Check sheet for the modelled part. Datum: model origin and axes. Units: mm. A direction names the side the tool comes from. Round coordinates to 2 decimals unless told otherwise and drop trailing zeros. Loops run counter-clockwise (first coordinate to the right, second up) from the corner with the lowest first, then second, coordinate; pieces in that order, holes last. Notation, with made-up numbers: (0.25, -32) -> (30.25, -32) arc R35 ccw to (30.25, 7) -> close; hole circle Ø2 at (42, 39). An arc over 180 degrees is marked (long way). One line per item, written item: value. Start each with the question number.
1. Go/stop test with flat-tipped pins: pin 1 (1.8 mm diameter, centred on x = 18, y = -3.5, fed in from +Z); pin 2 (10 mm diameter, centred on x = -5.5, y = 3.5, fed in from +Z); pin 3 (8 mm diameter, centred on x = 10.65, y = 0, fed in from +Z). Record where each tip stops, or that it passes through.
2. Cross-section at D-D on x = -10.65. Record the cut outline in (y, z), then the cut area to 3 significant figures.
3. Cross-section at C-C on z = 14. Record the cut outline in (x, y).
4. Material ranges on L1, parallel to Y at x = -10.65, z = -2.75; L2, parallel to Z at x = -4, y = 6.5; L3, parallel to Z at x = 13, y = 5.75, recorded low to high.
5. Set-up check for faces 4 (the face through (17, 0, 0)), 5 (the face through (-9.35, 0, 12)), 6 (the face through (-8.78, 0.14, 7.6)), 7 (the face through (-11.517, 3.905, -1.549)): record each of +Z, -Z, +X, -X, +Y, -Y from which the full face is reachable in a straight line by a thin tool's end or side.
6. Release check for a two-part mould opening along X. For faces 1 (the face through (-0.6, -0.14, -4.43)), 2 (the face through (-22, 0, 6)), 3 (the face through (4.85, 0, 8)) record: +X half, -X half, draft (parallel to the pull), parting line (faces both ways), or undercut.
from build123d import *

# Parameters (mm, degrees)
SKETCH_W        = 50
SKETCH_H        = 20
PAD_DEPTH       = 7
SKETCH001_W     = 11.6
SKETCH001_H     = 20
PAD001_DEPTH    = 1.2
SKETCH002_R     = 3.5
POCKET_DEPTH    = 8.201
SKETCH003_R     = 6
POCKET001_DEPTH = 1
CHAMFER_SIZE    = 2.49
SKETCH004_W     = 25
SKETCH004_H     = 20
PAD002_DEPTH    = 5
SKETCH005_R     = 4
POCKET002_DEPTH = 7
SKETCH006_W     = 15.65
SKETCH006_H     = 20
PAD003_DEPTH    = 10
POCKET003_DEPTH = 22.001
FILLET_R        = 2


with BuildPart() as part:
    # Sketch → Pad (new body)
    with BuildSketch(Plane.XY):
        Rectangle(SKETCH_W, SKETCH_H)
    extrude(amount=PAD_DEPTH)

    # Sketch001 (on Face6 of Pad) → Pad001 (join)
    with BuildSketch(Plane.XY.offset(7)):
        with Locations((10.65, 0)):
            Rectangle(SKETCH001_W, SKETCH001_H)
    extrude(amount=PAD001_DEPTH)

    # Sketch002 (on Face4 of Pad001) → Pocket (cut, through all)
    with BuildSketch(Plane(origin=(0, 0, 0), x_dir=(1, 0, 0), z_dir=(0, 0, -1))):
        with Locations((10.65, 0)):
            Circle(SKETCH002_R)
    extrude(amount=-POCKET_DEPTH, mode=Mode.SUBTRACT)

    # Sketch003 (on Face4 of Pocket) → Pocket001 (cut)
    with BuildSketch(Plane(origin=(0, 0, 0), x_dir=(1, 0, 0), z_dir=(0, 0, -1))):
        with Locations((10.65, 0)):
            Circle(SKETCH003_R)
    extrude(amount=-POCKET001_DEPTH, mode=Mode.SUBTRACT)

    # Chamfer
    chamfer_edges = [part.edges().sort_by_distance(p)[0] for p in [
        (7.15, 0, 1),
    ]]
    chamfer(chamfer_edges, length=CHAMFER_SIZE)

    # Sketch004 (on Face5 of Chamfer) → Pad002 (join)
    with BuildSketch(Plane(origin=(0, 0, 0), x_dir=(1, 0, 0), z_dir=(0, 0, -1))):
        with Locations((-12.5, 0)):
            Rectangle(SKETCH004_W, SKETCH004_H)
    extrude(amount=PAD002_DEPTH)

    # Sketch005 (on Face16 of Pad002) → Pocket002 (cut)
    with BuildSketch(Plane(origin=(0, 0, -5), x_dir=(1, 0, 0), z_dir=(0, 0, -1))):
        with Locations((-10.65, 0)):
            Circle(SKETCH005_R)
    extrude(amount=-POCKET002_DEPTH, mode=Mode.SUBTRACT)

    # Sketch006 (on Face20 of Pocket002) → Pad003 (join)
    with BuildSketch(Plane.XY.offset(7)):
        with Locations((-17.175, 0)):
            Rectangle(SKETCH006_W, SKETCH006_H)
    extrude(amount=PAD003_DEPTH)

    # Sketch007 (on Face16 of Pad003) → Pocket003 (cut, through all)
    with BuildSketch(Plane(origin=(0, 0, -5), x_dir=(1, 0, 0), z_dir=(0, 0, -1))):
        with BuildLine():
            ThreePointArc((-19.595918, 10), (-22, 0), (-19.595918, -10))
            Line((-19.595918, -10), (-25, -10))
            Line((-25, -10), (-25, 10))
            Line((-25, 10), (-19.595918, 10))
        make_face()
        with BuildLine():
            ThreePointArc((19.595918, -10), (22, 0), (19.595918, 10))
            Line((19.595918, 10), (25, 10))
            Line((25, 10), (25, -10))
            Line((25, -10), (19.595918, -10))
        make_face()
    extrude(amount=-POCKET003_DEPTH, mode=Mode.SUBTRACT)

    # Fillet
    fillet_edges = [part.edges().sort_by_distance(p)[0] for p in [
        (-22, 0, -5),
        (0, 0, -5),
        (0, 0, 0),
        (22, 0, 0),
        (22, 0, 7),
        (-9.35, 0, 17),
        (-22, 0, 17),
        (-9.35, 0, 7),
    ]]
    fillet(fillet_edges, radius=FILLET_R)


solid = part.part
Taken from the geometry:
1. pin 1: stops at z = 7
1. pin 2: stops at z = 16.81
1. pin 3: stops at z = 8.2
2. outline: (-10, -5) -> (-4, -5) -> (-4, 2) -> (4, 2) -> (4, -5) -> (10, -5) -> (10, 16.87) -> (-10, 16.87) -> close
2. area: 381 mm2
3. outline: (-19.6, -10) -> (-9.35, -10) -> (-9.35, 10) -> (-19.6, 10) arc R22 ccw to start
4. L1: y = -10 to -4, 4 to 10
4. L2: z = -5 to 7
4. L3: z = 0 to 8.2
5. face 4: -Z, +X, +Y, -Y
5. face 5: +Z, +X, +Y, -Y
5. face 6: +Z, +Y, -Y
5. face 7: -Z
6. face 1: +X half
6. face 2: -X half
6. face 3: undercut
